```python
from build123d import *

# Parameters (mm, degrees)
F1_DEPTH = 3.429


with BuildPart() as f1:
    # F0 (on Front) → F1 (new body)
    with BuildSketch(Plane.XZ):
        Polygon((-575.599027, 443.908663), (-575.599027, 461.688663), (-578.774027, 461.688663), (-578.774027, 503.598663), (-629.574027, 503.598663), (-629.574027, 461.688663), (-632.749027, 461.688663), (-632.749027, 443.908663), (-629.574027, 443.908663), (-629.574027, 401.998663), (-578.774027, 401.998663), (-578.774027, 443.908663), align=None)
        with BuildLine():
            Line((-594.649027, 471.848663), (-594.649027, 433.748663))
            ThreePointArc((-594.649027, 433.748663), (-604.174027, 424.223663), (-613.699027, 433.748663))
            Line((-613.699027, 433.748663), (-613.699027, 471.848663))
            ThreePointArc((-613.699027, 471.848663), (-604.174027, 481.373663), (-594.649027, 471.848663))
        make_face(mode=Mode.SUBTRACT)
    extrude(amount=F1_DEPTH)


solid = f1.part
```
Verification items for the finished model (mm, model axes). A direction names the side the tool comes from. Coordinates: 2 decimals unless noted, no trailing zeros. Loops run counter-clockwise (first coordinate to the right, second up) from the corner with the lowest first, then second, coordinate; pieces in that order, holes last. Notation, with made-up numbers: (34.5, 74.5) -> (42.5, 74.5) arc R26 ccw to (42.5, 95.5) -> close; hole circle Ø11 at (-37, 9). An arc over 180 degrees is marked (long way). Answer in a Markdown table with one row per item.
1) Section check B-B (z = 445.5). Record the cut outline in (x, y).
The answers:
| item | result |
|---|---|
| outline | (-632.75, -3.43) -> (-613.7, -3.43) -> (-613.7, 0) -> (-632.75, 0) -> close; (-594.65, -3.43) -> (-575.6, -3.43) -> (-575.6, 0) -> (-594.65, 0) -> close |
2) Access from +Z, -Z, +X, -X, +Y, -Y to the whole of each face (thin tool, end or side, straight path). Record for faces 5 (the face through (-613.699, -2, 453)), 6 (the face through (-629.574, -2, 423)), 7 (the face through (-577, -2, 443.909)), 8 (the face through (-577, -2, 461.689)), 9 (the face through (-631, -2, 461.689)).
The answers:
| item | result |
|---|---|
| face 5 | +Y, -Y |
| face 6 | -Z, -X, +Y, -Y |
| face 7 | -Z, +X, +Y, -Y |
| face 8 | +Z, +X, +Y, -Y |
| face 9 | +Z, -X, +Y, -Y |
3) Section check C-C (x = -600). Record the cut outline in (y, z).
The answers:
| item | result |
|---|---|
| outline | (-3.43, 402) -> (0, 402) -> (0, 425.19) -> (-3.43, 425.19) -> close; (-3.43, 480.41) -> (0, 480.41) -> (0, 503.6) -> (-3.43, 503.6) -> close |
4) Section check A-A (y = -2.8). Record the cut outline in (x, z) (3 decimals).
The answers:
| item | result |
|---|---|
| outline | (-632.749, 443.909) -> (-629.574, 443.909) -> (-629.574, 401.999) -> (-578.774, 401.999) -> (-578.774, 443.909) -> (-575.599, 443.909) -> (-575.599, 461.689) -> (-578.774, 461.689) -> (-578.774, 503.599) -> (-629.574, 503.599) -> (-629.574, 461.689) -> (-632.749, 461.689) -> close; hole (-613.699, 433.749) arc R9.525 ccw to (-594.649, 433.749) -> (-594.649, 471.849) arc R9.525 ccw to (-613.699, 471.849) -> close |
5) Draft check along X on faces 1 (the face through (-603.965, -1.69, 424.226)), 2 (the face through (-629.574, -2, 483)), 3 (the face through (-592, -3.429, 454)), 4 (the face through (-575.599, -2, 453)). Enter one of: released by +X, released by -X, zero draft, split by the parting line, or undercut.
The answers:
| item | result |
|---|---|
| face 1 | undercut |
| face 2 | released by -X |
| face 3 | zero draft |
| face 4 | released by +X |
6) Scan lines: line 1 along X through (y, z) = (-1.5, 439.5); line 2 along X through (y, z) = (-1.45, 495); line 3 along Z through (x, y) = (-608.5, -0.2). Record each from-to range of solid material in increasing order. Write a range as from..to.
The answers:
| item | result |
|---|---|
| line 1 | x = -629.57..-613.7, -594.65..-578.77 |
| line 2 | x = -629.57..-578.77 |
| line 3 | z = 402..425.26, 480.33..503.6 |
7) Depth check by flat-ended pin: P1, Ø1, axis at x = -632, y = -2.5, coming from the -Z side; P2, Ø1, axis at y = -2, z = 418.5, coming from the -X side; P3, Ø1.6, axis at x = -632, y = -1.5, coming from the +Z side. Enter the tip coordinate at first touch or a pass-through.
The answers:
| item | result |
|---|---|
| P1 | stops at z = 443.91 |
| P2 | stops at x = -629.57 |
| P3 | stops at z = 461.69 |
